Geometry: see drawing. Coordinates: mm, zero at the bounding-box minimum. A direction names the side the tool comes from. Coordinates: 2 decimals unless noted, no trailing zeros. Order: outer loops, then holes, each group sorted by start corner. A loop starts at its lowest first (then second) coordinate and runs counter-clockwise, first axis right, second up. Notation, with made-up numbers: (-9, 76) - (46, 76) arc R21 ccw to (46, 92) - close; hole circle Ø5 at (64, 88.5). An arc over 180 degrees is marked (long way). Use a Markdown table: item, result. Add a question column.
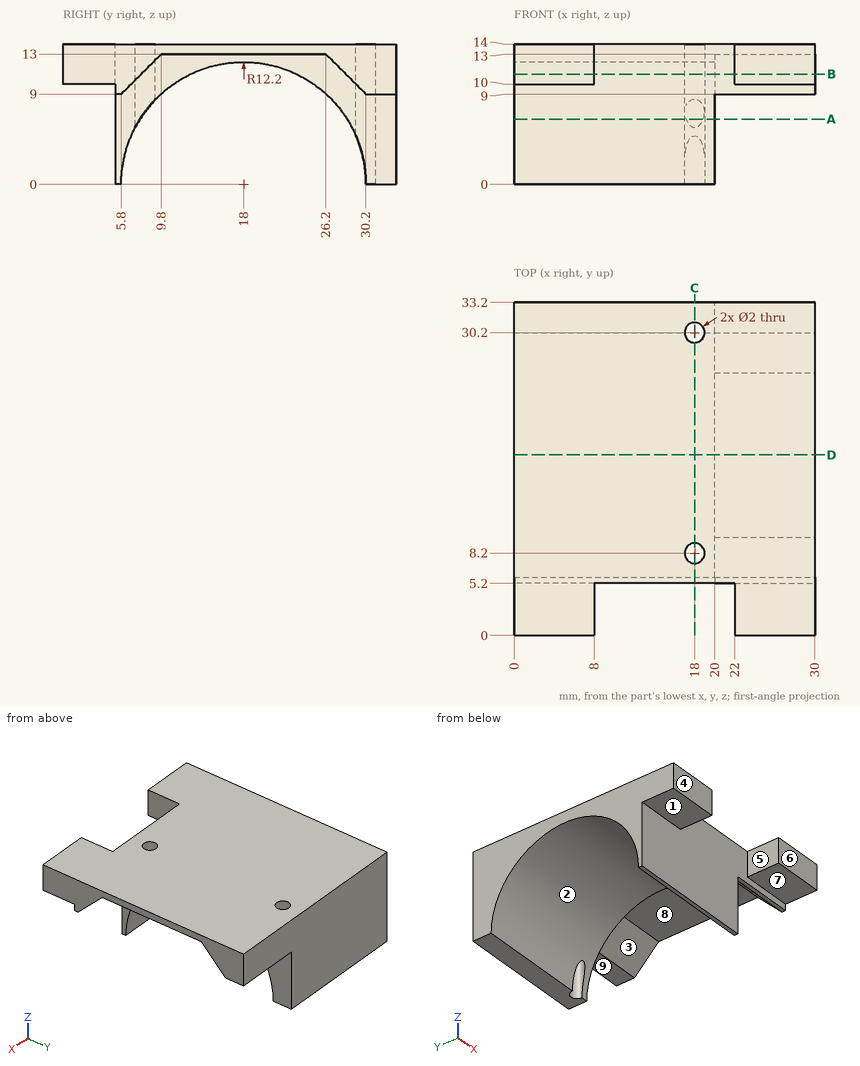
1) Pull-direction query (Y, two-part tool) for the marked faces 1, 2, 3 and 4; classes: pulls with the +Y half, pulls with the -Y half, needs draft (parallel to the pull), parting line crosses it, or undercut.
2) Cut plane B-B (z = 11). Return the cut outline in (x, y), and give its area (3 significant figures).
3) Cut plane C-C (x = 18). Return the cut outline in (y, z), and give its area (3 significant figures).
4) Reachability of the marked faces 5, 6, 7, 8 and 9 from +Z, -Z, +X, -X, +Y, -Y: full face, straight path, thin tool, end or side. Return the list, or none.
5) Contact query for flat-ended pins moving along their axis: P1, Ø7, axis at x = 21, z = 5.5, coming from the -Y side; P2, Ø1.5, axis at y = 22.5, z = 11.5, coming from the +X side; P3, Ø5.5, axis at x = 25, y = 3.5, coming from the -Z side; P4, Ø1.6, axis at x = 18, y = 30.2, coming from the -Z side. Output: stop coordinate, or through.
6) Material intervals for L1, parallel to X at y = 30.2, z = 5.5; L2, parallel to Y at x = 18, z = 8; L3, parallel to Y at x = 18, z = 10.75, sorted ascending.
7) Cut plane A-A (z = 6.5). Return the cut outline in (x, y), and give its area (3 significant figures).
8) Cut plane D-D (y = 18). Return the cut outline in (x, z), and give its area (3 significant figures).
Computed:
| question | item | result |
|---|---|---|
| 1 | face 1 | needs draft |
| 1 | face 2 | undercut |
| 1 | face 3 | undercut |
| 1 | face 4 | pulls with the -Y half |
| 2 | outline | (0, 0) - (8, 0) - (8, 5.2) - (22, 5.2) - (22, 0) - (30, 0) - (30, 7.8) - (20, 7.8) - (20, 12.72) - (0, 12.72) - close; (0, 23.28) - (20, 23.28) - (20, 28.2) - (30, 28.2) - (30, 33.2) - (0, 33.2) - close; hole circle Ø2 at (18, 8.2); hole circle Ø2 at (18, 30.2) |
| 2 | area | 502 mm2 |
| 3 | outline | (5.2, 0) - (5.8, 0) arc R12.2 cw to (7.2, 5.67) - (7.2, 14) - (5.2, 14) - close; (9.2, 8.45) arc R12.2 cw to (29.2, 4.84) - (29.2, 14) - (9.2, 14) - close; (31.2, 0) - (33.2, 0) - (33.2, 14) - (31.2, 14) - close |
| 3 | area | 120 mm2 |
| 4 | face 5 | +Z, -Z, -Y |
| 4 | face 6 | +Z, -Z, +X, -X, -Y |
| 4 | face 7 | -Z, +X, -X, -Y |
| 4 | face 8 | -Z, +X |
| 4 | face 9 | -Z, +X, +Y, -Y |
| 5 | P1 | stops at y = 5.2 |
| 5 | P2 | stops at x = 20 |
| 5 | P3 | stops at z = 9 |
| 5 | P4 | passes through |
| 6 | L1 | x = 0 to 17, 19 to 20 |
| 6 | L2 | y = 5.2 to 7.2, 27.21 to 29.2, 31.2 to 33.2 |
| 6 | L3 | y = 5.2 to 7.2, 9.2 to 12.23, 23.77 to 29.2, 31.2 to 33.2 |
| 7 | outline | (0, 5.2) - (20, 5.2) - (20, 7.68) - (18.85, 7.68) arc R1 cw to (17.15, 7.68) - (0, 7.68) - close; (0, 28.32) - (20, 28.32) - (20, 33.2) - (0, 33.2) - close; hole circle Ø2 at (18, 30.2) |
| 7 | area | 143 mm2 |
| 8 | outline | (0, 12.2) - (20, 12.2) - (20, 13) - (30, 13) - (30, 14) - (0, 14) - close |
| 8 | area | 46.0 mm2 |
